from build123d import *

# Parameters (mm, degrees)
SKETCH1_W           = 50.6476
SKETCH1_H           = 5.4102
SKETCH1_R           = 3.175
BOSS_EXTRUDE1_DEPTH = 5.4102


with BuildPart() as part:
    # Sketch1 → Boss-Extrude1 (new body)
    with BuildSketch(Plane(origin=(0, 0, 0), x_dir=(1, 0, 0), z_dir=(0, 1, 0))):
        Polygon((-190.881, 47.5361), (-190.881, -72.9361), (165.481, -72.9361), (165.481, -47.5361), (114.8334, -47.5361), (114.8334, -42.1259), (165.481, -42.1259), (165.481, 47.5361), (62.5475, 47.5361), (62.5475, -42.1259), (63.7286, -42.1259), (63.7286, -47.5361), (-63.7286, -47.5361), (-63.7286, -42.1259), (-73.30694, -42.1259), (-73.30694, 47.5361), align=None)
        with Locations((-140.1572, -44.831)):
            Rectangle(SKETCH1_W, SKETCH1_H, mode=Mode.SUBTRACT)
        with Locations(Location((-181.229, 34.8361, 0), (0, 0, 270))):
            Circle(SKETCH1_R, mode=Mode.SUBTRACT)
        with Locations(Location((152.781, -60.2361, 0), (0, 0, 270))):
            Circle(SKETCH1_R, mode=Mode.SUBTRACT)
        with Locations(Location((-178.181, -60.2361, 0), (0, 0, 270))):
            Circle(SKETCH1_R, mode=Mode.SUBTRACT)
        with Locations(Location((136.271, -60.2361, 0), (0, 0, 270))):
            Circle(SKETCH1_R, mode=Mode.SUBTRACT)
        with Locations(Location((-155.829, 34.8361, 0), (0, 0, 270))):
            Circle(SKETCH1_R, mode=Mode.SUBTRACT)
        with Locations(Location((-86.00694, 34.8361, 0), (0, 0, 270))):
            Circle(SKETCH1_R, mode=Mode.SUBTRACT)
        with Locations(Location((145.06956, 34.8361, 0), (0, 0, 270))):
            Circle(SKETCH1_R, mode=Mode.SUBTRACT)
        with Locations(Location((75.2475, 34.8361, 0), (0, 0, 270))):
            Circle(SKETCH1_R, mode=Mode.SUBTRACT)
    extrude(amount=BOSS_EXTRUDE1_DEPTH)


solid = part.part
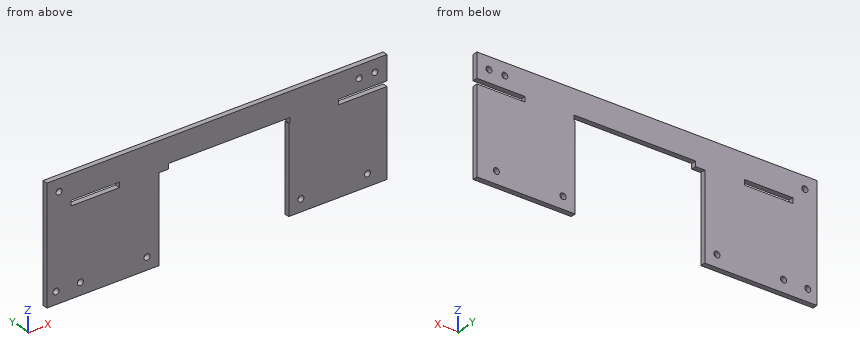
Geometry: final body of the model. Coordinates: model frame, mm. Give positions to 0.01 mm unless a question says otherwise; leave off trailing zeros. Write each loop counter-clockwise with the first axis right and the second up, starting at its lowest first coordinate (ties: lowest second). Pieces come first, ordered by that corner, then holes.
(1) Ray query, line 1 (Z direction, x = 145, y = 2.35); line 2 (Z direction, x = 120, y = 0.85); line 3 (X direction, y = 5, z = 31). Return the intervals inside material, ascending.
(2) First-contact query: P1, Ø4, axis at x = -181.23, z = -34.84, coming from the +Y side; P2, Ø2, axis at x = 27.5, y = 5, coming from the -Z side. Flat tips, straight axial feed; report the tip coordinate or a pass-through.
(3) Cut plane C-C, the plane y = 3.8. Give the number of separate pieces and of enclosed holes in the cut face, then the cut area to 3 significant figures.
(4) Cut plane B-B, the plane z = 22. Return loops of the section in (x, y), then the cut area to 3 significant figures.
(5) Cut plane D-D, the plane x = 27.5. Return loops of the section in (y, z), then the cut area to 3 significant figures.
(6) Cut plane A-A, the plane x = -143.5. Return loops of the section in (y, z), then the cut area to 3 significant figures.
Values follow:
1. line 1: z = -47.54 to -38.01, -31.66 to 42.13, 47.54 to 72.94
1. line 2: z = -47.54 to 42.13, 47.54 to 72.94
1. line 3: x = -190.88 to -73.31, 62.55 to 165.48
2. P1: passes through
2. P2: stops at z = 47.54
3. separate pieces: 1
3. enclosed holes: 9
3. area: 29,300 mm2
4. outline: (-190.88, 0) - (-73.31, 0) - (-73.31, 5.41) - (-190.88, 5.41) - close; (62.55, 0) - (165.48, 0) - (165.48, 5.41) - (62.55, 5.41) - close
4. area: 1,190 mm2
5. outline: (0, 47.54) - (5.41, 47.54) - (5.41, 72.94) - (0, 72.94) - close
5. area: 137 mm2
6. outline: (0, -47.54) - (5.41, -47.54) - (5.41, 42.13) - (0, 42.13) - close; (0, 47.54) - (5.41, 47.54) - (5.41, 72.94) - (0, 72.94) - close
6. area: 623 mm2
